CAD build for the part. Positions are in the model's coordinates, mm. Round coordinates to 2 decimals unless told otherwise and drop trailing zeros. Write each loop counter-clockwise with the first axis right and the second up, starting at its lowest first coordinate (ties: lowest second). Pieces come first, ordered by that corner, then holes. Notation, with made-up numbers: (83, -5.75) - (141, -5.75) arc R21 ccw to (141, 1.25) - close; hole circle Ø9 at (89, 47.25). An arc over 180 degrees is marked (long way). Use one line per item in the form item = value. Start each with the question number.
Item 1: Band-saw the part on C-C, the plane z = 1.4. List the corners of the cut face in (x, y).
Item 2: Drill centre lines: L1, parallel to Y at x = 0, z = -0.8; L2, parallel to X at y = -2.5, z = 0.6; L3, parallel to Y at x = 3.5, z = -1.6. Where is each one in solid material? Low to high.
Item 3: Band-saw the part on B-B, the plane y = 3.5. List the corners of the cut face in (x, z).
Item 4: Band-saw the part on D-D, the plane x = -10.75. List the corners of the cut face in (y, z), and give its area (3 significant figures).
Item 5: Pull direction Y, two halves, no side cores. Call faces 1 (the flat face through (-6, -9, 2)), 2 (the flat face through (10.172, 5.764, 0.028)), 3 (the cylindrical face through (-2.17, -9.76, -0.03)): +Y half, -Y half, draft (parallel to the pull), parting line (faces both ways), or undercut.
Item 6: Band-saw the part on A-A, the plane x = 0. List the corners of the cut face in (y, z).
from build123d import *

# Parameters (mm, degrees)
SKETCH1_R           = 10
BOSS_EXTRUDE1_DEPTH = 2


with BuildPart() as part:
    # Sketch1 → Boss-Extrude1 (new, symmetric)
    with BuildSketch(Plane.XY):
        Polygon((6.75, -11.691342951), (13.5, 0), (6.75, 11.691342951), (-6.75, 11.691342951), (-13.5, 0), (-6.75, -11.691342951), align=None)
        Circle(SKETCH1_R, mode=Mode.SUBTRACT)
    extrude(amount=BOSS_EXTRUDE1_DEPTH, both=True)

    # Sketch4 → Cut-Revolve1 (revolve, cut)
    with BuildSketch(Plane(origin=(0, 0, 0), x_dir=(1, 0, 0), z_dir=(0, 1, 0))):
        Polygon((-13.5, 2), (-12.5, 2), (-13.5, 1), align=None)
    cut_revolve1 = revolve(axis=Axis((0, 0, -2), (0, 0, 1)), mode=Mode.SUBTRACT)

    # Mirror1: Cut-Revolve1 across plane
    add(cut_revolve1.mirror(Plane.XY), mode=Mode.SUBTRACT)


solid = part.part
Determined:
q1.outline = (-13.08, -0.73) - (-7.17, -10.96) arc R13.1 ccw to (-5.91, -11.69) - (5.91, -11.69) arc R13.1 ccw to (7.17, -10.96) - (13.08, -0.73) arc R13.1 ccw to (13.08, 0.73) - (7.17, 10.96) arc R13.1 ccw to (5.91, 11.69) - (-5.91, 11.69) arc R13.1 ccw to (-7.17, 10.96) - (-13.08, 0.73) arc R13.1 ccw to start; hole circle Ø20 at (0, 0)
q2.L1 = -11.69 to -10, 10 to 11.69
q2.L2 = -12.06 to -9.68, 9.68 to 12.06
q2.L3 = -11.69 to -9.37, 9.37 to 11.69
q3.outline = (-11.48, -2) - (-9.37, -2) - (-9.37, 2) - (-11.48, 2) - close; (9.37, -2) - (11.48, -2) - (11.48, 2) - (9.37, 2) - close
q4.outline = (-4.76, -2) - (4.76, -2) - (4.76, 2) - (-4.76, 2) - close
q4.area = 38.1 mm²
q5.face_1 = draft
q5.face_2 = +Y half
q5.face_3 = undercut
q6.outline = (-11.69, -2) - (-10, -2) - (-10, 2) - (-11.69, 2) - close; (10, -2) - (11.69, -2) - (11.69, 2) - (10, 2) - close
